Geometry: final body of the model. Coordinates: model frame, mm. Give positions to 0.01 mm unless a question says otherwise; leave off trailing zeros. Answer as a JSON object with one key per item and string values.
from build123d import *

# Parameters (mm, degrees)
SKETCH1_W             = 280
SKETCH1_H             = 12
BOSS_EXTRUDE1_DEPTH   = 33
LPATTERN1_COUNT       = 9
LPATTERN1_PITCH       = 15
LPATTERN1_COL_COUNT   = 9
LPATTERN1_COL_PITCH   = 15
M4_TAPPED_HOLE1_D     = 3.3
M4_TAPPED_HOLE1_DEPTH = 15
M4_TAPPED_HOLE1_TIP   = 0.991420021


with BuildPart() as part:
    # Sketch1 → Boss-Extrude1 (new body)
    with BuildSketch(Plane(origin=(0, 0, 0), x_dir=(1, 0, 0), z_dir=(0, 1, 0))):
        Rectangle(SKETCH1_W, SKETCH1_H)
    extrude(amount=BOSS_EXTRUDE1_DEPTH)

    # Sketch4 → M2 Tapped Hole1 (revolve, cut)
    with BuildSketch(Plane(origin=(0, 33, 0), x_dir=(0, 0, 1), z_dir=(1, 0, 0))):
        Polygon((0, 0), (0, 15.480688495), (0.8, 15), (0.8, 0), align=None)
    m2_tapped_hole1 = revolve(axis=Axis((0, 39.35, 0), (0, -1, 0)), mode=Mode.SUBTRACT)

    # LPattern1: M2 Tapped Hole1 ×9
    with Locations(*[(i * LPATTERN1_PITCH, 0, 0) for i in range(1, LPATTERN1_COUNT)]):
        add(m2_tapped_hole1, mode=Mode.SUBTRACT)

    # LPattern1 col: M2 Tapped Hole1 ×9
    with Locations(*[(-i * LPATTERN1_COL_PITCH, 0, 0) for i in range(1, LPATTERN1_COL_COUNT)]):
        add(m2_tapped_hole1, mode=Mode.SUBTRACT)

    # M4 Tapped Hole1
    with Locations(Plane(origin=(0, 0, 0), x_dir=(-1, 0, 0), z_dir=(0, -1, 0))):
        with Locations((-120, 0), (120, 0)):
            Hole(M4_TAPPED_HOLE1_D / 2, depth=M4_TAPPED_HOLE1_DEPTH)
            with Locations((0, 0, -(M4_TAPPED_HOLE1_DEPTH + M4_TAPPED_HOLE1_TIP / 2))):  # 118° drill point
                Cone(0, M4_TAPPED_HOLE1_D / 2, M4_TAPPED_HOLE1_TIP, mode=Mode.SUBTRACT)


solid = part.part
1) Line query: line 1 (Z direction, x = -45, y = 28.75). Output: solid intervals per line, ascending. Write a range as from..to.
Geometry check:
{"line 1": "z = -6..-0.8, 0.8..6"}
2) Pull-direction query (X, two-part tool) for faces 1 (the flat face through (140, 16, 0)), 2 (the flat face through (-140, 16, 0)), 3 (the flat face through (-2, 16, -6)); classes: pulls with the +X half, pulls with the -X half, needs draft (parallel to the pull), parting line crosses it, or undercut.
Geometry check:
{"face 1": "pulls with the +X half", "face 2": "pulls with the -X half", "face 3": "needs draft"}
3) Contact query for flat-ended pins moving along their axis: P1, Ø1.3, axis at x = 105, z = 0, coming from the +Y side; P2, Ø2.5, axis at x = 120, z = 0, coming from the -Y side; P3, Ø1, axis at x = 0, z = 0, coming from the +Y side. Output: stop coordinate, or through.
Geometry check:
{"P1": "stops at y = 17.91", "P2": "stops at y = 15.24", "P3": "stops at y = 17.82"}
